```python
from build123d import *

# Parameters (mm, degrees)
BOSS_EXTRU_1_DEPTH            = 50
DIAM_TRE_DU_PER_AGE_3_0_3_1_D = 3


with BuildPart() as part:
    # Esquisse1 → Boss.-Extru.1 (new body)
    with BuildSketch(Plane.XY):
        with BuildLine():
            ThreePointArc((-26.998355192, 6.25), (-28, 0), (-26.998355192, -6.25))
            ThreePointArc((-26.998355192, -6.25), (0, -24.5), (26.998355192, -6.25))
            ThreePointArc((26.998355192, -6.25), (28, 0), (26.998355192, 6.25))
            ThreePointArc((26.998355192, 6.25), (0, 24.5), (-26.998355192, 6.25))
        make_face()
    extrude(amount=BOSS_EXTRU_1_DEPTH)

    # Diamètre du perçage Ø3.0 (3)1 (through all)
    with Locations(Plane.XY.offset(50)):
        with Locations((0, 12.5), (0, -12.5)):
            Hole(DIAM_TRE_DU_PER_AGE_3_0_3_1_D / 2)


solid = part.part
```
Could you check a few things on this model? Use its own coordinates, in mm. Give positions to 0.01 mm unless a question says otherwise; leave off trailing zeros. Loops run counter-clockwise (first coordinate to the right, second up) from the corner with the lowest first, then second, coordinate; pieces in that order, holes last. Notation, with made-up numbers: (35.5, 15.25) - (43.5, 15.25) arc R33 cw to (43.5, 47.25) - close; hole circle Ø10 at (55.5, -37). An arc over 180 degrees is marked (long way). Answer in a Markdown table with one row per item. Add a question column.
Q1. We'd pull the mould along X, two halves only. Please class faces 1 (the face through (0, 0, 0)), 2 (the face through (-0.484, -24.496, 24.65)), 3 (the face through (0, -14, 25)): +X half, -X half, draft (parallel to the pull), parting line (faces both ways), or undercut.
Q2. If we section it at D-D (x = -9.5): List the corners of the cut face in (y, z) for me, plus the area to 3 significant figures.
Q3. If we section it at A-A (z = 43.5): List the corners of the cut face in (x, y) for me, plus the area to 3 significant figures.
Q4. If we section it at B-B (x = 0): List the corners of the cut face in (y, z) for me, plus the area to 3 significant figures.
Q5. For pin 1 (12 mm diameter, centred on x = 11.5, y = -8.5, fed in from -Z); pin 2 (6 mm diameter, centred on x = 13.5, z = 23.5, fed in from +Y); pin 3 (1.5 mm diameter, centred on x = 12.5, z = 30, fed in from -Y); pin 4 (10 mm diameter, centred on x = 13.5, z = 39, fed in from -Y), each with a flat end and sliding along its axis, tell me the tip position at first contact or that it passes through.
Q6. If we section it at C-C (y = -12.5): List the corners of the cut face in (x, z) for me, plus the area to 3 significant figures.
Q7. Please list where these lines run through material, in increasing order: L1, parallel to X at y = 12, z = 21; L2, parallel to X at y = -10, z = 13.5; L3, parallel to Y at x = -10, z = 24.5. Write a range as from..to.
The answers:
| question | item | result |
|---|---|---|
| 1 | face 1 | draft |
| 1 | face 2 | parting line |
| 1 | face 3 | undercut |
| 2 | outline | (-22.91, 0) - (22.91, 0) - (22.91, 50) - (-22.91, 50) - close |
| 2 | area | 2,290 mm^2 |
| 3 | outline | (-27, -6.25) arc R29.1 ccw to (27, -6.25) arc R20 ccw to (27, 6.25) arc R29.1 ccw to (-27, 6.25) arc R20 ccw to start; hole circle Ø3 at (0, -12.5); hole circle Ø3 at (0, 12.5) |
| 3 | area | 2,100 mm^2 |
| 4 | outline | (-24.5, 0) - (-14, 0) - (-14, 50) - (-24.5, 50) - close; (-11, 0) - (11, 0) - (11, 50) - (-11, 50) - close; (14, 0) - (24.5, 0) - (24.5, 50) - (14, 50) - close |
| 4 | area | 2,150 mm^2 |
| 5 | pin 1 | stops at z = 0 |
| 5 | pin 2 | stops at y = 22.54 |
| 5 | pin 3 | stops at y = -22.02 |
| 5 | pin 4 | stops at y = -23.23 |
| 6 | outline | (-23.54, 0) - (-1.5, 0) - (-1.5, 50) - (-23.54, 50) - close; (1.5, 0) - (23.54, 0) - (23.54, 50) - (1.5, 50) - close |
| 6 | area | 2,200 mm^2 |
| 7 | L1 | x = -23.9..-1.41, 1.41..23.9 |
| 7 | L2 | x = -25.17..25.17 |
| 7 | L3 | y = -22.73..22.73 |
